Read the model definition and answer for the solid it produces. Units are mm, in the model's axes. A direction names the side the tool comes from. Coordinates: 2 decimals unless noted, no trailing zeros. Order: outer loops, then holes, each group sorted by start corner. A loop starts at its lowest first (then second) coordinate and runs counter-clockwise, first axis right, second up. Notation, with made-up numbers: (-1, -5) -> (27, -5) arc R13 ccw to (27, 15) -> close; hole circle Ø5 at (82, 3). An arc over 180 degrees is marked (long way). Use CSV: the item, a comma, the result in double quotes.
```python
from build123d import *

# Parameters (mm, degrees)
CROQUIS2_W              = 30
CROQUIS2_H              = 10
CORTAR_EXTRUIR1_DEPTH   = 64
CROQUIS3_W              = 60
CROQUIS3_H              = 25.4
CROQUIS3_R              = 3.2
SALIENTE_EXTRUIR1_DEPTH = 6.4


with BuildPart() as part:
    # Croquis1 → Revolución1 (revolve)
    with BuildSketch(Plane.XY, mode=Mode.PRIVATE) as revoluci_n1_sk:
        Polygon((-8, 55), (-10.5, 55), (-10.5, 60), (-16, 60), (-16, 0), (-10.5, 0), (-10.5, 5), (-8, 5), align=None)
    revolve(revoluci_n1_sk.sketch.rotate(Axis((0, 0, 0), (0, 1, 0)), 270), axis=Axis((0, 0, 0), (0, 1, 0)))

    # Croquis2 → Cortar-Extruir1 (cut)
    with BuildSketch(Plane.XZ):
        with Locations((0, -19)):
            Rectangle(CROQUIS2_W, CROQUIS2_H)
    extrude(amount=-CORTAR_EXTRUIR1_DEPTH, mode=Mode.SUBTRACT)

    # Croquis3 → Saliente-Extruir1 (add)
    with BuildSketch(Plane(origin=(0, 0, -14), x_dir=(-1, 0, 0), z_dir=(0, 0, -1))):
        with Locations((0, 30)):
            Rectangle(CROQUIS3_W, CROQUIS3_H)
        with Locations((-22, 36.7)):
            Circle(CROQUIS3_R, mode=Mode.SUBTRACT)
        with Locations((-22, 23.3)):
            Circle(CROQUIS3_R, mode=Mode.SUBTRACT)
        with Locations((22, 36.7)):
            Circle(CROQUIS3_R, mode=Mode.SUBTRACT)
        with Locations((22, 23.3)):
            Circle(CROQUIS3_R, mode=Mode.SUBTRACT)
    extrude(amount=SALIENTE_EXTRUIR1_DEPTH)


solid = part.part
```
Item 1: Straight lines are drawn through the part: line 1 along Y through (x, z) = (-22, -18); line 2 along X through (y, z) = (36.5, -17); line 3 along Z through (x, y) = (14, 32). For each, find the intervals that lie inside material, in ascending order.
Return value:
line 1,"y = 17.3 to 20.1, 26.5 to 33.5, 39.9 to 42.7"
line 2,"x = -30 to -25.19, -18.81 to 18.81, 25.19 to 30"
line 3,"z = -20.4 to -14, -7.75 to 7.75"
Item 2: Each of these flat-tipped pins is pushed along its axis until it touches: P1, Ø6, axis at x = -17.5, z = -10.5, coming from the +Y side; P2, Ø5, axis at x = 2, y = 8.5, coming from the -Z side; P3, Ø10, axis at x = 22, y = 36.7, coming from the +Z side; P4, Ø5, axis at x = 16, y = 47, coming from the -Z side. Where does it stop, or does it pass through?
Return value:
P1,"passes through"
P2,"stops at z = -14"
P3,"stops at z = -14"
P4,"stops at z = -8.59"
Item 3: Find section C-C, the plane z = 1. Give the vertices of the cut face in (x, y).
Return value:
outline,"(-15.97, 0) -> (-10.45, 0) -> (-10.45, 5) -> (-7.94, 5) -> (-7.94, 55) -> (-10.45, 55) -> (-10.45, 60) -> (-15.97, 60) -> close; (7.94, 5) -> (10.45, 5) -> (10.45, 0) -> (15.97, 0) -> (15.97, 60) -> (10.45, 60) -> (10.45, 55) -> (7.94, 55) -> close"
Item 4: Find section A-A, the plane y = 36.7. Give the vertices of the cut face in (x, z).
Return value:
outline,"(-30, -20.4) -> (-25.2, -20.4) -> (-25.2, -14) -> (-30, -14) -> close; (-18.8, -20.4) -> (18.8, -20.4) -> (18.8, -14) -> (7.75, -14) arc R16 ccw (long way) to (-7.75, -14) -> (-18.8, -14) -> close; (25.2, -20.4) -> (30, -20.4) -> (30, -14) -> (25.2, -14) -> close; hole circle Ø16 at (0, 0)"
Item 5: The mould has two halves that part along Z. Classify faces 1 (the flat face through (0, 9, -14)), 2 (the cylindrical face through (-0.59, 29.58, 15.99)), 3 (the cylindrical face through (-3.2, 2.5, -10)), 4 (the cylindrical face through (25.2, 23.4, -17.2)): +Z half, -Z half, draft (parallel to the pull), parting line (faces both ways), or undercut.
Return value:
face 1,"-Z half"
face 2,"undercut"
face 3,"undercut"
face 4,"draft"
Item 6: A tool of negligible diameter and unlimited length cuts with its end or side. For faces 5 (the flat face through (0, 17.3, -17)), 6 (the cylindrical face through (-3.2, 57.5, -10)), 7 (the flat face through (8, 5, 2)), 8 (the flat face through (-19, 30, -14)), from which of +Z, -Z, +X, -X, +Y, -Y can it reach the whole face along a straight path? Write none if from no direction.
Return value:
face 5,"-Z, +X, -X, -Y"
face 6,"+Y"
face 7,"-Y"
face 8,"-X, +Y, -Y"
Item 7: Find section B-B, the plane x = -22. Give the vertices of the cut face in (y, z).
Return value:
outline,"(17.3, -20.4) -> (20.1, -20.4) -> (20.1, -14) -> (17.3, -14) -> close; (26.5, -20.4) -> (33.5, -20.4) -> (33.5, -14) -> (26.5, -14) -> close; (39.9, -20.4) -> (42.7, -20.4) -> (42.7, -14) -> (39.9, -14) -> close"
Item 8: Find section D-D, the plane x = -5.5. Give the vertices of the cut face in (y, z).
Return value:
outline,"(0, -14) -> (17.3, -14) -> (17.3, -20.4) -> (42.7, -20.4) -> (42.7, -14) -> (60, -14) -> (60, -8.94) -> (55, -8.94) -> (55, -5.81) -> (5, -5.81) -> (5, -8.94) -> (0, -8.94) -> close; (0, 8.94) -> (5, 8.94) -> (5, 5.81) -> (55, 5.81) -> (55, 8.94) -> (60, 8.94) -> (60, 15.02) -> (0, 15.02) -> close"
